from build123d import *

# Parameters (mm, degrees)
SKETCH1_W               = 113
SKETCH1_H               = 75
SKETCH1_W_2             = 98
SKETCH1_H_2             = 63
BOSS_EXTRUDE1_DEPTH     = 3
FILLET1_R               = 4
SKETCH2_W               = 98
SKETCH2_H               = 2.5
BOSS_EXTRUDE2_DEPTH     = 3
FILLET2_R               = 1.5
SKETCH3_W               = 98
SKETCH3_H               = 63
SKETCH3_W_2             = 90
SKETCH3_H_2             = 60
BOSS_EXTRUDE3_DEPTH     = 1
CUT_EXTRUDE1_DEPTH      = 114.169815067
CUT_EXTRUDE1_DEPTH_BACK = 114.169815067


with BuildPart() as part:
    # Sketch1 → Boss-Extrude1 (new body)
    with BuildSketch(Plane.XY):
        with Locations((-26.020950744, 3.343078266)):
            Rectangle(SKETCH1_W, SKETCH1_H)
        with Locations((-26.020950744, 3.343078266)):
            Rectangle(SKETCH1_W_2, SKETCH1_H_2, mode=Mode.SUBTRACT)
    extrude(amount=BOSS_EXTRUDE1_DEPTH)

    # Fillet1
    fillet1_edges = [part.edges().sort_by_distance(p)[0] for p in [
        (-82.520950744, 40.843078266, 1.5),
        (30.479049256, 40.843078266, 1.5),
        (30.479049256, -34.156921734, 1.5),
        (-82.520950744, -34.156921734, 1.5),
    ]]
    fillet(fillet1_edges, radius=FILLET1_R)

    # Sketch2 → Boss-Extrude2 (add)
    with BuildSketch(Plane(origin=(0, 0, 0), x_dir=(-1, 0, 0), z_dir=(0, 0, -1))):
        with Locations((26.020950744, 36.093078266)):
            Rectangle(SKETCH2_W, SKETCH2_H)
        with Locations((26.020950744, -29.406921734)):
            Rectangle(SKETCH2_W, SKETCH2_H)
    extrude(amount=BOSS_EXTRUDE2_DEPTH)

    # Fillet2
    fillet2_edges = [part.edges().sort_by_distance(p)[0] for p in [
        (-82.520950744, 3.343078266, 3),
        (-26.020950744, 40.843078266, 3),
        (-26.020950744, -34.156921734, 3),
        (30.479049256, 3.343078266, 3),
        (29.307476381, 39.67150539, 3),
        (29.307476381, -32.985348859, 3),
        (-81.349377868, -32.985348859, 3),
        (-81.349377868, 39.67150539, 3),
    ]]
    fillet(fillet2_edges, radius=FILLET2_R)

    # Sketch3 → Boss-Extrude3 (add)
    with BuildSketch(Plane.XY.offset(3)):
        with Locations((-26.020950744, 3.343078266)):
            Rectangle(SKETCH3_W, SKETCH3_H)
        with Locations((-26.020950744, 3.343078266)):
            Rectangle(SKETCH3_W_2, SKETCH3_H_2, mode=Mode.SUBTRACT)
    extrude(amount=-BOSS_EXTRUDE3_DEPTH)

    # Sketch4 → Cut-Extrude1 (cut, two sides: drawn at the far end of the back side and taken through both)
    with BuildSketch(Plane.ZY.offset(75.020950744).offset(-CUT_EXTRUDE1_DEPTH_BACK)):
        Polygon((0, 37.343078266), (-2.5, 34.843078266), (-3, 34.843078266), (-3, 37.343078266), align=None)
    extrude(amount=CUT_EXTRUDE1_DEPTH + CUT_EXTRUDE1_DEPTH_BACK, mode=Mode.SUBTRACT)


solid = part.part
The listing builds one solid part. Answer for the finished solid, in the listing's coordinates (mm). A direction names the side the tool comes from. Give positions to 0.01 mm unless a question says otherwise; leave off trailing zeros. Write each loop counter-clockwise with the first axis right and the second up, starting at its lowest first coordinate (ties: lowest second). Pieces come first, ordered by that corner, then holes. Notation, with made-up numbers: (-37.75, -8.75) -> (-11.75, -8.75) arc R23 ccw to (-11.75, 30.25) -> close; hole circle Ø2 at (85.25, 65). An arc over 180 degrees is marked (long way). One line per question, with ' | ' between items. Start each with the question number.
1. Section C-C (z = -1.5) is taken. Determine the outline of the cut face in (x, y), plus the area to 3 significant figures.
2. Find the intervals of material crossed by probe 1 along Y at (x, z) = (-15, 1.65); probe 2 along X at (y, z) = (11, 0.25); probe 3 along Y at (x, z) = (-57.5, 1), in increasing order.
3. Section D-D (x = 21.5) is taken. Determine the outline of the cut face in (y, z).
4. Section B-B (y = -8) is taken. Determine the outline of the cut face in (x, z), plus the area to 3 significant figures.
5. Given pin 1 Ø0.8 at (y, z) = (0.5, 2.5) entering from +X; pin 2 Ø2.5 at (x, z) = (-9.5, -1.5) entering from -Y; pin 3 Ø1.2 at (y, z) = (-29.5, -2) entering from +X, each flat-ended and moving along its own axis, determine where each tip first touches the part or whether it passes through.
6. Section A-A (x = -16) is taken. Determine the outline of the cut face in (y, z).
7. For faces 1 (the flat face through (-75.021, 36, -1)), 2 (the flat face through (-25, -30.657, -1)), 3 (the flat face through (-30, -27, 2)), 4 (the flat face through (22.979, -29, -1)), 5 (the flat face through (-25.335, 36.111, -1.233)), determine the directions among +Z, -Z, +X, -X, +Y, -Y from which every point of the face is accessible in a straight line to the end or side of a thin tool.
Response values:
1) outline: (-75.02, -30.66) -> (22.98, -30.66) -> (22.98, -28.16) -> (-75.02, -28.16) -> close; (-75.02, 34.84) -> (22.98, 34.84) -> (22.98, 35.84) -> (-75.02, 35.84) -> close | area: 343 mm2
2) probe 1: -34.15 to -28.16, 34.84 to 40.84 | probe 2: -82.52 to -75.02, 22.98 to 30.48 | probe 3: -34.16 to -28.16, 34.84 to 40.84
3) outline: (-34.16, 0) -> (-30.66, 0) -> (-30.66, -3) -> (-28.16, -3) -> (-28.16, 2) -> (34.84, 2) -> (34.84, -2.5) -> (37.34, 0) -> (40.84, 0) -> (40.84, 1.5) arc R1.5 ccw to (39.34, 3) -> (-32.66, 3) arc R1.5 ccw to (-34.16, 1.5) -> close
4) outline: (-82.52, 0) -> (-75.02, 0) -> (-75.02, 2) -> (-71.02, 2) -> (-71.02, 3) -> (-81.02, 3) arc R1.5 ccw to (-82.52, 1.5) -> close; (18.98, 2) -> (22.98, 2) -> (22.98, 0) -> (30.48, 0) -> (30.48, 1.5) arc R1.5 ccw to (28.98, 3) -> (18.98, 3) -> close | area: 52.0 mm2
5) pin 1: x = 30.35 | pin 2: y = -30.66 | pin 3: x = 22.98
6) outline: (-34.16, 0) -> (-30.66, 0) -> (-30.66, -3) -> (-28.16, -3) -> (-28.16, 2) -> (-26.66, 2) -> (-26.66, 3) -> (-32.66, 3) arc R1.5 ccw to (-34.16, 1.5) -> close; (33.34, 2) -> (34.84, 2) -> (34.84, -2.5) -> (37.34, 0) -> (40.84, 0) -> (40.84, 1.5) arc R1.5 ccw to (39.34, 3) -> (33.34, 3) -> close
7) face 1: -Z, -X, +Y, -Y | face 2: -Z, +X, -X, -Y | face 3: -Z | face 4: -Z, +X, +Y, -Y | face 5: -Z, +X, -X, +Y
